```python
from build123d import *

# Parameters (mm, degrees)
F0_W     = 56.4
F0_H     = 56.4
F1_DEPTH = 80
F2_R     = 19.05
F3_DEPTH = 1.6
F4_R     = 4
F5_DEPTH = 19.4
F6_R     = 2
F7_DEPTH = 25
F8_R     = 26
F9_DEPTH = 25
F10_R    = 3
F11_R    = 2


with BuildPart() as f1:
    # F0 (on Top) → F1 (new body)
    with BuildSketch(Plane.XY):
        Rectangle(F0_W, F0_H)
    extrude(amount=F1_DEPTH)

    # F2 (on face) → F3 (join)
    with BuildSketch(Plane.XY.offset(80)):
        Circle(F2_R)
    extrude(amount=F3_DEPTH)

    # F4 (on face) → F5 (join)
    with BuildSketch(Plane.XY.offset(81.6)):
        Circle(F4_R)
    extrude(amount=F5_DEPTH)

    # F6 (on face) → F7 (cut)
    with BuildSketch(Plane.XY.offset(80)):
        with Locations((23.55, 23.55)):
            Circle(F6_R)
        with Locations((-23.55, 23.55)):
            Circle(F6_R)
        with Locations((-23.55, -23.55)):
            Circle(F6_R)
        with Locations((23.55, -23.55)):
            Circle(F6_R)
    extrude(amount=-F7_DEPTH, mode=Mode.SUBTRACT)

    # F8 (on face) → F9 (join)
    with BuildSketch(Plane(origin=(0, 0, 0), x_dir=(1, 0, 0), z_dir=(0, 0, -1))):
        Circle(F8_R)
    extrude(amount=F9_DEPTH)

    # F10
    f10_edges = [f1.edges().sort_by_distance(p)[0] for p in [
        (0, -28.2, 0),
    ]]
    fillet(f10_edges, radius=F10_R)

    # F11
    f11_edges = [f1.edges().sort_by_distance(p)[0] for p in [
        (-26, 0, -25),
    ]]
    fillet(f11_edges, radius=F11_R)


solid = f1.part
```
The listing builds one solid part. Answer for the finished solid, in the listing's coordinates (mm). A direction names the side the tool comes from. Round coordinates to 2 decimals unless told otherwise and drop trailing zeros. Loops run counter-clockwise (first coordinate to the right, second up) from the corner with the lowest first, then second, coordinate; pieces in that order, holes last.
Q1. Find the intervals of material crossed by line 1 (Y direction, x = -23.55, z = 68.5); line 2 (Z direction, x = -4, y = 23); line 3 (Z direction, x = -3.5, y = -8), in increasing order.
Q2. Given pin 1 Ø3 at (x, y) = (-23.55, -23.55) entering from -Z; pin 2 Ø3.5 at (x, y) = (23.55, 23.55) entering from +Z; pin 3 Ø2 at (x, y) = (-18, 20.5) entering from +Z, each flat-ended and moving along its own axis, determine where each tip first touches the part or whether it passes through.
Q3. Section B-B, the plane z = -14.5 is taken. Determine the outline of the cut face in (x, y), then the cut area to 3 significant figures.
Q4. For a pull along X with two mould halves and no side action, classify faces 1 (the face through (-28.2, 0, 39)), 2 (the face through (0, 5, 81.6)), 3 (the face through (-21.703, -24.316, 67.675)) as released by +X, released by -X, zero draft, split by the parting line, or undercut.
Q5. Section A-A, the plane y = 0 is taken. Determine the outline of the cut face in (x, z), then the cut area to 3 significant figures.
Q6. Which of the six approach directions +Z, -Z, +X, -X, +Y, -Y give full straight-line access (tool end or side, diameter ignored) to faces 4 (the face through (-17.15, -27.34, 0.9)), 5 (the face through (17.45, -27.34, 0.9)), 6 (the face through (0, 28.2, 39)), 7 (the face through (-20.633, 15.821, -11.339)), 8 (the face through (24, 24, 55))?
Completed:
1. line 1: y = -28.2 to -25.55, -21.55 to 21.55, 25.55 to 28.2
1. line 2: z = -25 to 80
1. line 3: z = -25 to 81.6
2. pin 1: stops at z = 0
2. pin 2: stops at z = 55
2. pin 3: stops at z = 80
3. outline: circle Ø52 at (0, 0)
3. area: 2,120 mm2
4. face 1: released by -X
4. face 2: zero draft
4. face 3: undercut
5. outline: (-28.2, 0) - (-26, 0) - (-26, -23) arc R2 ccw to (-24, -25) - (24, -25) arc R2 ccw to (26, -23) - (26, 0) - (28.2, 0) - (28.2, 80) - (19.05, 80) - (19.05, 81.6) - (4, 81.6) - (4, 101) - (-4, 101) - (-4, 81.6) - (-19.05, 81.6) - (-19.05, 80) - (-28.2, 80) - close
5. area: 6,030 mm2
6. face 4: -Z, -X, -Y
6. face 5: -Z, +X, -Y
6. face 6: +Z, -Z, +X, -X, +Y
6. face 7: -Z
6. face 8: +Z
